Part model, mm, in its own coordinate system. Coordinates: 2 decimals unless noted, no trailing zeros. Loops run counter-clockwise (first coordinate to the right, second up) from the corner with the lowest first, then second, coordinate; pieces in that order, holes last. Notation, with made-up numbers: (50.5, 0) -> (91.5, 0) arc R15 ccw to (91.5, 9) -> close; hole circle Ø9 at (68.25, 86). An arc over 180 degrees is marked (long way). One line per question, with ' | ' between items. Start each with the question number.
1) Cut at D-D (y = 0.4). List the corners of the cut face in (x, z), plus the area to 3 significant figures.
2) Probe L1, parallel to X at y = 0.2, z = 0; L2, parallel to Z at x = 7.25, y = -0.5. List the from-to ranges inside material, lowest first. Write a range as from..to.
3) Two-plate mould, pull along Y, no slides. Class faces 1 (the face through (1, -0.622, 10)), 2 (the face through (10, 0.622, 1)), 3 (the face through (0.31, -0.01, 10.33)): released by +Y, released by -Y, zero draft, split by the parting line, or undercut.
4) Cut at B-B (z = 2.25). List the corners of the cut face in (x, y).
5) Cut at C-C (x = 0). List the corners of the cut face in (y, z).
6) Cut at A-A (x = -5.75). List the corners of the cut face in (y, z), plus the area to 3 significant figures.
from build123d import *

# Parameters (mm, degrees)
SKETCH3_R                = 11.0998
SKETCH3_R_2              = 9.7536
BOSS_EXTRUDE1_DEPTH      = 0.6223
BOSS_EXTRUDE1_DEPTH_BACK = 0.6223
CUT_EXTRUDE1_DEPTH       = 12.0998


with BuildPart() as part:
    # Sketch3 → Boss-Extrude1 (new body, two sides)
    with BuildSketch(Plane(origin=(0, 0, 0), x_dir=(1, 0, 0), z_dir=(0, 1, 0))) as boss_extrude1_sk:
        Circle(SKETCH3_R)
        Circle(SKETCH3_R_2, mode=Mode.SUBTRACT)
    extrude(amount=BOSS_EXTRUDE1_DEPTH)
    extrude(boss_extrude1_sk.sketch, amount=-BOSS_EXTRUDE1_DEPTH_BACK)

    # Sketch4 → Cut-Extrude1 (cut, through all)
    with BuildSketch(Plane.XY):
        Polygon((2.838309027, 1.280985718), (-2.9315561, -1.050191113), (-2.838309027, -1.280985718), (2.9315561, 1.050191113), align=None)
    extrude(amount=CUT_EXTRUDE1_DEPTH, mode=Mode.SUBTRACT)


solid = part.part
Reported:
1) outline: (0.66, 9.73) -> (0.66, 11.08) arc R11.1 ccw (long way) to (1.32, 11.02) -> (1.32, 9.66) arc R9.75 cw (long way) to start | area: 87.3 mm²
2) L1: x = -11.1..-9.75, 9.75..11.1 | L2: z = -8.4..-6.52, 6.52..8.4
3) face 1: released by -Y | face 2: released by +Y | face 3: undercut
4) outline: (-10.87, -0.62) -> (-9.49, -0.62) -> (-9.49, 0.62) -> (-10.87, 0.62) -> close; (9.49, -0.62) -> (10.87, -0.62) -> (10.87, 0.62) -> (9.49, 0.62) -> close
5) outline: (-0.62, -11.1) -> (0.62, -11.1) -> (0.62, -9.75) -> (-0.62, -9.75) -> close; (-0.62, 9.75) -> (-0.13, 9.75) -> (-0.13, 11.1) -> (-0.62, 11.1) -> close; (0.13, 9.75) -> (0.62, 9.75) -> (0.62, 11.1) -> (0.13, 11.1) -> close
6) outline: (-0.62, -9.49) -> (0.62, -9.49) -> (0.62, -7.88) -> (-0.62, -7.88) -> close; (-0.62, 7.88) -> (0.62, 7.88) -> (0.62, 9.49) -> (-0.62, 9.49) -> close | area: 4.02 mm²
